The model under review builds one solid part; all positions refer to its coordinate system, in mm. A direction names the side the tool comes from. Give positions to 0.01 mm unless a question says otherwise; leave off trailing zeros. Loops run counter-clockwise (first coordinate to the right, second up) from the corner with the lowest first, then second, coordinate; pieces in that order, holes last. Notation, with made-up numbers: (-36.5, 22) - (-28.5, 22) arc R25 cw to (-28.5, 58) - close; hole circle Ø8 at (68.25, -39). An arc over 180 degrees is marked (long way). Answer as a JSON object with one key per item and string values.
from build123d import *

# Parameters (mm, degrees)
F0_R     = 11
F0_R_2   = 5.5
F1_DEPTH = 2.5
F0_R_3   = 4.1
F2_DEPTH = 3.3
F3_DEPTH = 6.05
F4_R     = 2.49999


# Not quite as in the source:
# - a fillet or chamfer is up to 0.001 mm smaller than in the source, because OpenCascade refuses the exact size


with BuildPart() as f1:
    # F0 (on Top) → F1 (new body)
    with BuildSketch(Plane.XY):
        Circle(F0_R)
        Circle(F0_R_2, mode=Mode.SUBTRACT)
    extrude(amount=F1_DEPTH)

    # F0 (on Top) → F2 (join, through all)
    with BuildSketch(Plane.XY):
        Circle(F0_R_2)
        Circle(F0_R_3, mode=Mode.SUBTRACT)
    extrude(amount=F2_DEPTH)

    # F0 (on Top) → F3 (join, through all)
    with BuildSketch(Plane.XY):
        Circle(F0_R_3)
    extrude(amount=F3_DEPTH)

    # F4 (radius 2.5 in the source; OpenCascade refuses exactly that, so slightly less here)
    f4_edges = [f1.edges().sort_by_distance(p)[0] for p in [
        (-11, 0, 0),
    ]]
    fillet(f4_edges, radius=F4_R)


solid = f1.part
Q1. Consider section C-C, the plane z = 0.5. State the section outline as (x, y) points, plus the area to 3 significant figures.
Results:
{"outline": "circle Ø20 at (0, 0)", "area": "314 mm^2"}
Q2. Consider section D-D, the plane z = 4.5. State the section outline as (x, y) points.
Results:
{"outline": "circle Ø8.2 at (0, 0)"}
Q3. Clearance check with flat-ended pins moving along their axes: pin 1 Ø1 at (x, y) = (-8, 1) entering from +Z; pin 2 Ø6 at (x, y) = (6, 2) entering from -Z. State where each tip first meets the part, or that it passes through.
Results:
{"pin 1": "stops at z = 2.5", "pin 2": "stops at z = 0"}
Q4. To check wall thickness, follow probe 1 along Z at (x, y) = (6.25, -0.75); probe 2 along X at (y, z) = (2.5, 4.75); probe 3 along Y at (x, z) = (2, 3). State the ranges of each line that lie inside material, in increasing order. Write a range as [from, to].
Results:
{"probe 1": "z = [0, 2.5]", "probe 2": "x = [-3.25, 3.25]", "probe 3": "y = [-5.12, 5.12]"}
Q5. For faces 1 (the face through (0, 0, 6.05)), 2 (the face through (-3, 5, 2.5)), list the 3-axis set-ups (+Z, -Z, +X, -X, +Y, -Y) from which the entire face can be reached by the end or side of a thin tool; tool diameter is ignored.
Results:
{"face 1": "+Z, +X, -X, +Y, -Y", "face 2": "+Z"}
